from build123d import *

# Parameters (mm, degrees)
SKETCH2_W           = 120
SKETCH2_H           = 105
SKETCH2_R           = 1.4
BOSS_EXTRUDE2_DEPTH = 5
CUT_EXTRUDE7_DEPTH  = 90.336442732
FILLET5_R           = 10
SKETCH10_R          = 20
CUT_EXTRUDE9_DEPTH  = 90.336442732
CHAMFER3_SIZE       = 3
FILLET6_R           = 5
CHAMFER4_SIZE       = 1
SKETCH11_R          = 2.15
CUT_EXTRUDE10_DEPTH = 90.336442732
SKETCH13_R          = 3.25
CUT_EXTRUDE12_DEPTH = 2.5


with BuildPart() as part:
    # Sketch2 → Boss-Extrude2 (new body)
    with BuildSketch(Plane(origin=(0, 0, 0), x_dir=(1, 0, 0), z_dir=(0, 1, 0))):
        with Locations((0, 13.5)):
            Rectangle(SKETCH2_W, SKETCH2_H)
        with Locations(Location((-28, -28, 0), (0, 0, 270))):
            Circle(SKETCH2_R, mode=Mode.SUBTRACT)
        with Locations(Location((28, -28, 0), (0, 0, 270))):
            Circle(SKETCH2_R, mode=Mode.SUBTRACT)
        with Locations(Location((20, 42, 0), (0, 0, 270))):
            Circle(SKETCH2_R, mode=Mode.SUBTRACT)
        with Locations(Location((-20, 42, 0), (0, 0, 270))):
            Circle(SKETCH2_R, mode=Mode.SUBTRACT)
    extrude(amount=BOSS_EXTRUDE2_DEPTH)

    # Sketch9 → Cut-Extrude7 (cut, through all)
    with BuildSketch(Plane(origin=(0, 5, 0), x_dir=(1, 0, 0), z_dir=(0, 1, 0))):
        with BuildLine():
            Line((-17.474873734, -34.025126266), (-23.449747468, -40))
            Line((-23.449747468, -40), (23.449747468, -40))
            Line((23.449747468, -40), (17.474873734, -34.025126266))
            ThreePointArc((17.474873734, -34.025126266), (16.339392013, -33.266421636), (15, -33))
            Line((15, -33), (-15, -33))
            ThreePointArc((-15, -33), (-16.339392013, -33.266421636), (-17.474873734, -34.025126266))
        make_face()
    extrude(amount=-CUT_EXTRUDE7_DEPTH, mode=Mode.SUBTRACT)

    # Fillet5
    fillet5_edges = [part.edges().sort_by_distance(p)[0] for p in [
        (-60, 2.5, -66),
        (60, 2.5, -66),
        (60, 2.5, 39),
        (-60, 2.5, 39),
    ]]
    fillet(fillet5_edges, radius=FILLET5_R)

    # Sketch10 → Cut-Extrude9 (cut, through all)
    with BuildSketch(Plane(origin=(0, 0, 0), x_dir=(1, 0, 0), z_dir=(0, 1, 0))):
        with Locations(Location((0, 0, 0), (0, 0, 270))):
            Circle(SKETCH10_R)
    extrude(amount=CUT_EXTRUDE9_DEPTH, mode=Mode.SUBTRACT)

    # Chamfer3
    chamfer3_edges = [part.edges().sort_by_distance(p)[0] for p in [
        (0, 5, -20),
    ]]
    chamfer(chamfer3_edges, length=CHAMFER3_SIZE)

    # Fillet6
    fillet6_edges = [part.edges().sort_by_distance(p)[0] for p in [
        (-22.449747468, 2.5, 39),
        (22.449747468, 2.5, 39),
    ]]
    fillet(fillet6_edges, radius=FILLET6_R)

    # Chamfer4
    chamfer4_edges = [part.edges().sort_by_distance(p)[0] for p in [
        (16.339392013, 5, 33.266421636),
        (0, 5, 33),
        (-16.339392013, 5, 33.266421636),
        (-19.230077554, 5, 35.780330086),
        (-60, 5, -13.5),
        (0, 5, -66),
        (60, 5, -13.5),
        (-37.26040764, 5, 39),
        (-57.071067812, 5, 36.071067812),
        (57.071067812, 5, 36.071067812),
        (57.071067812, 5, -63.071067812),
        (-57.071067812, 5, -63.071067812),
        (19.230077554, 5, 35.780330086),
        (37.26040764, 5, 39),
        (22.607398118, 5, 38.619397663),
        (-22.607398118, 5, 38.619397663),
    ]]
    chamfer(chamfer4_edges, length=CHAMFER4_SIZE)

    # Sketch11 → Cut-Extrude10 (cut, through all)
    with BuildSketch(Plane(origin=(0, 5, 0), x_dir=(1, 0, 0), z_dir=(0, 1, 0))):
        with Locations(Location((-50, 56, 0), (0, 0, 270))):
            Circle(SKETCH11_R)
        with Locations(Location((50, 56, 0), (0, 0, 270))):
            Circle(SKETCH11_R)
        with Locations(Location((-50, -19, 0), (0, 0, 270))):
            Circle(SKETCH11_R)
        with Locations(Location((50, -19, 0), (0, 0, 270))):
            Circle(SKETCH11_R)
    extrude(amount=-CUT_EXTRUDE10_DEPTH, mode=Mode.SUBTRACT)

    # Sketch13 → Cut-Extrude12 (cut)
    with BuildSketch(Plane.XZ):
        with Locations(Location((-28, 28, 0), (0, 0, 270))):
            Circle(SKETCH13_R)
        with Locations(Location((28, 28, 0), (0, 0, 270))):
            Circle(SKETCH13_R)
        with Locations(Location((-20, -42, 0), (0, 0, 270))):
            Circle(SKETCH13_R)
        with Locations(Location((20, -42, 0), (0, 0, 270))):
            Circle(SKETCH13_R)
    extrude(amount=-CUT_EXTRUDE12_DEPTH, mode=Mode.SUBTRACT)


solid = part.part
Build history of the part. All positions in model axes, mm. A direction names the side the tool comes from. Round coordinates to 2 decimals unless told otherwise and drop trailing zeros. Write each loop counter-clockwise with the first axis right and the second up, starting at its lowest first coordinate (ties: lowest second). Pieces come first, ordered by that corner, then holes. Notation, with made-up numbers: M 1,-1.5 L 56,-1.5 A15 cw 56,8.5 Z; hole C 71.5,86 d6. An arc over 180 degrees is marked long. Answer in a Markdown table with one row per item.
1. Mould opens along X. For faces 6 (the face through (37, 2, 39)), 7 (the face through (51.81, 2.54, 20.16)), 8 (the face through (56.415, 4.826, -62.558)) say: +X half, -X half, draft (parallel to the pull), parting line (faces both ways), or undercut.
Geometry check:
| item | result |
|---|---|
| face 6 | draft |
| face 7 | undercut |
| face 8 | +X half |
2. Flat gauge pins, fed straight in: P1, Ø6, axis at x = 28, z = 28, coming from the -Y side; P2, Ø5, axis at x = 20, z = -42, coming from the +Y side; P3, Ø1.2, axis at x = -6, y = 2, coming from the +Z side. Where does each tip first touch, or does it go through?
Geometry check:
| item | result |
|---|---|
| P1 | y = 2.5 |
| P2 | y = 5 |
| P3 | z = 33 |
3. Saw through at B-B (z = -42). List the corners of the cut face in (x, y).
Geometry check:
| item | result |
|---|---|
| outline | M -60,0 L -23.25,0 L -23.25,2.5 L -21.4,2.5 L -21.4,5 L -59,5 L -60,4 Z; M -18.6,2.5 L -16.75,2.5 L -16.75,0 L 16.75,0 L 16.75,2.5 L 18.6,2.5 L 18.6,5 L -18.6,5 Z; M 21.4,2.5 L 23.25,2.5 L 23.25,0 L 60,0 L 60,4 L 59,5 L 21.4,5 Z |
4. Saw through at C-C (y = 1.15). State how many separate pieces and enclosed holes the cut face has, and give its area (3 significant figures).
Geometry check:
| item | result |
|---|---|
| separate pieces | 1 |
| enclosed holes | 9 |
| area | 10,800 mm2 |
5. Saw through at A-A (x = 0). List the corners of the cut face in (y, z), and give its area (3 significant figures).
Geometry check:
| item | result |
|---|---|
| outline | M 0,-66 L 4,-66 L 5,-65 L 5,-23 L 2,-20 L 0,-20 Z; M 0,20 L 2,20 L 5,23 L 5,32 L 4,33 L 0,33 Z |
| area | 285 mm2 |
6. Probe L1, parallel to X at y = 3.65, z = -42; L2, parallel to X at y = 1.3, z = -56; L3, parallel to X at y = 3.6, z = 19. List the from-to ranges inside material, lowest first. Write a range as [from, to].
Geometry check:
| item | result |
|---|---|
| L1 | [-60, -21.4], [-18.6, 18.6], [21.4, 60] |
| L2 | [-60, -52.15], [-47.85, 47.85], [52.15, 60] |
| L3 | [-60, -52.15], [-47.85, -10.27], [10.27, 47.85], [52.15, 60] |
7. Which spindle directions (+Z, -Z, +X, -X, +Y, -Y) get a long thin tool onto all of the face, cutting with end or side? Do faces 1 (the face through (19.46, 3.73, -40.71)), 2 (the face through (19.25, 2.03, 35.8)), 3 (the face through (-56.558, 4.826, -62.415)), 4 (the face through (-19.55, 4.49, 35.41)), 5 (the face through (25.117, 1.232, 26.5)). Say none if no direction does.
Geometry check:
| item | result |
|---|---|
| face 1 | +Y, -Y |
| face 2 | +Z, +Y, -Y |
| face 3 | -Z, -X, +Y |
| face 4 | +Z, +Y |
| face 5 | -Y |
